```python
from build123d import *

# Parameters (mm, degrees)
F0_R     = 77.47
F1_DEPTH = 2.54
F3_T     = -1.27


# Not quite as in the source:
# - a fillet or chamfer that OpenCascade refuses, or shapes differently, is made with other operations: its cross-section is extruded or revolved along the edge and cut away or added
# - a feature names something its author has since deleted; it is built from what else it names


with BuildPart() as f1:
    # F0 (on Front) → F1 (new body)
    with BuildSketch(Plane.XZ):
        Circle(F0_R)
    extrude(amount=F1_DEPTH)

    # F2: fillet of radius 7.62 on 1 edges, made by hand

    # F2_s1 → F2_t2 (revolve, cut)
    with BuildSketch(Plane.XY):
        with BuildLine():
            ThreePointArc((77.47, -2.54), (74.9012393105, -0.6639235197), (71.7903873372, 0))
            Line((71.7903873372, 0), (77.47, 0))
            Line((77.47, 0), (77.47, -2.54))
        make_face()
    revolve(axis=Axis((0, 0, 0), (0, -1, 0)), mode=Mode.SUBTRACT)

    # F3
    f3_openings = [f1.faces().sort_by_distance(p)[0] for p in [
        (0, -2.54, 0),
    ]]
    offset(amount=F3_T, openings=f3_openings)


solid = f1.part
```
Could you check a few things on this model? Use its own coordinates, in mm. Round coordinates to 2 decimals unless told otherwise and drop trailing zeros. Write each loop counter-clockwise with the first axis right and the second up, starting at its lowest first coordinate (ties: lowest second). Pieces come first, ordered by that corner, then holes.
(1) Suppose I cut it at A-A on y = -2.05. Write out the boundary of the cut face in (x, z), and give its area (3 significant figures).
Findings below:
outline: circle Ø153.98 at (0, 0); hole circle Ø149.68 at (0, 0)
area: 1,030 mm2
(2) For pin 1 (1 mm diameter, centred on x = 32.5, y = -2, fed in from +Z); pin 2 (10 mm diameter, centred on x = 28, z = 51, fed in from -Y), each with a flat end and sliding along its axis, tell me the tip position at first contact or that it passes through.
Findings below:
pin 1: stops at z = 70.33
pin 2: stops at y = -1.27
(3) Thinking about a two-plate mould opening in X: for faces 1 (the face through (-1, -1.27, 1)), 2 (the face through (17, -2.54, -74)), which applies, +X half, -X half, draft (parallel to the pull), parting line (faces both ways), or undercut?
Findings below:
face 1: undercut
face 2: draft
(4) If I drill on probe 1 along Y at (x, z) = (-21, -63); probe 2 along Z at (x, y) = (0.5, -2.25); probe 3 along X at (y, z) = (-2.2, -36), over which ranges is the centre line in solid material (lowest first)?
Findings below:
probe 1: y = -1.27 to 0
probe 2: z = -77.2 to -75.18, 75.18 to 77.2
probe 3: x = -68.23 to -65.91, 65.91 to 68.23
